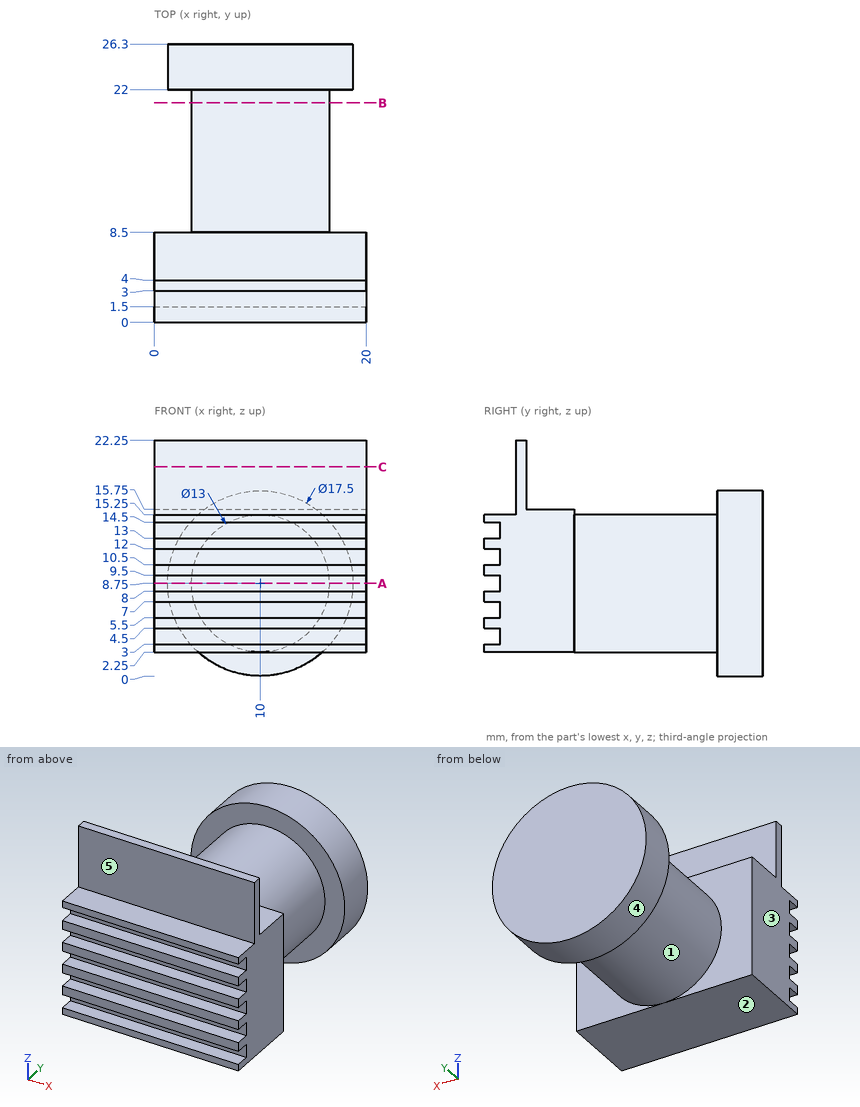
Study the drawing (mm; zero at the part's minimum x, y, z) and answer. A direction names the side the tool comes from. Give positions to 0.01 mm unless a question says otherwise; leave off trailing zeros. Loops run counter-clockwise (first coordinate to the right, second up) from the corner with the lowest first, then second, coordinate; pieces in that order, holes last. Notation, with made-up numbers: (79, 2) -> (85, 2) arc R17 cw to (85, 14) -> close; hole circle Ø10 at (2, 43). An arc over 180 degrees is marked (long way). Write item = value, one per line. Start each with the question number.
(1) Find section C-C on z = 19.75. Give the vertices of the cut face in (x, y), and give its area (3 significant figures).
(2) Which of the six approach directions +Z, -Z, +X, -X, +Y, -Y give full straight-line access (tool end or side, diameter ignored) to the marked faces 1, 2, 3, 4 and 5?
(3) Find the intervals of material crossed by probe 1 along Y at (x, z) = (5, 13.25); probe 2 along Y at (x, z) = (6.75, 20.75); probe 3 along Y at (x, z) = (7, 4), in increasing order. Write a range as from..to.
(4) Find section B-B on y = 20.75. Give the vertices of the cut face in (x, z), and give its area (3 significant figures).
(5) Find section A-A on z = 8.75. Give the vertices of the cut face in (x, y), and give its area (3 significant figures).
(6) Given pin 1 Ø2 at (y, z) = (21.5, 5) entering from -X; pin 2 Ø5.5 at (x, z) = (10.5, 18.5) entering from -Y; pin 3 Ø2 at (y, z) = (21.5, 12) entering from +X, each flat-ended and moving along its own axis, determine where each tip first touches the part or whether it passes through.
From the geometry:
q1.outline = (0, 3) -> (20, 3) -> (20, 4) -> (0, 4) -> close
q1.area = 20.0 mm^2
q2.face_1 = none
q2.face_2 = -Z, +X, -X, -Y
q2.face_3 = +Z, -Z, -X, +Y, -Y
q2.face_4 = +Y
q2.face_5 = +Z, +X, -X, -Y
q3.probe_1 = 1.5..8.5, 22..26.3
q3.probe_2 = 3..4
q3.probe_3 = 1.5..26.3
q4.outline = circle Ø13 at (10, 8.75)
q4.area = 133 mm^2
q5.outline = (0, 1.5) -> (20, 1.5) -> (20, 8.5) -> (16.5, 8.5) -> (16.5, 22) -> (18.75, 22) -> (18.75, 26.3) -> (1.25, 26.3) -> (1.25, 22) -> (3.5, 22) -> (3.5, 8.5) -> (0, 8.5) -> close
q5.area = 391 mm^2
q6.pin_1 = 1.74
q6.pin_2 = 3
q6.pin_3 = 18.42
